Geometry check sheet. Reference: the model listing, model coordinates, mm. A direction names the side the tool comes from. Give positions to 0.01 mm unless a question says otherwise; leave off trailing zeros. Loops run counter-clockwise (first coordinate to the right, second up) from the corner with the lowest first, then second, coordinate; pieces in that order, holes last.
1. Cross-section at B-B, the plane y = 0. State how many separate pieces and enclosed holes the cut face has, plus the area to 3 significant figures.
2. Material ranges on L1, parallel to Y at x = 7.5, z = 0; L2, parallel to X at y = 0, z = 2.6; L3, parallel to Y at x = 17.25, z = 0, recorded low to high.
3. Cross-section at A-A, the plane x = 16.5. Record the cut outline in (y, z), plus the area to 3 significant figures.
4. Tool access check on faces 1 (the cylindrical face through (16.7, -3.6, 2.8)), 2 (the conical face through (8.226, 5.081, 5.134)), 3 (the cylindrical face through (10.046, 0.596, 2.919)). Record the directions out of +Z, -Z, +X, -X, +Y, -Y that give a thin tool (end or side, any length) a straight path to the whole face; none if there is none.
5. Go/stop test with flat-tipped pins: pin 1 Ø1 at (y, z) = (-4, -2.5) entering from +X; pin 2 Ø3 at (x, z) = (3.5, 2) entering from +Y. Record where each tip stops, or that it passes through.
from build123d import *

# Parameters (mm, degrees)
SKETCH3_W          = 1.5748
SKETCH3_H          = 4.5593
HOLE1_D            = 3.2512
HOLE1_DEPTH        = 21.463
HOLE1_CSINK_D      = 4.0132
HOLE1_CSINK_ANGLE  = 90
SKETCH6_W          = 25.4
SKETCH6_H          = 25.4
SKETCH6_W_2        = 12.7
SKETCH6_H_2        = 12.7
CUT_EXTRUDE1_DEPTH = 21.463
HOLE2_D            = 3.96748
HOLE2_DEPTH        = 6.35
HOLE2_CSINK_D      = 4.826
HOLE2_CSINK_ANGLE  = 90


with BuildPart() as part:
    # Sketch1 → Revolve1 (revolve)
    with BuildSketch(Plane.XY):
        Polygon((0, 0), (0, 4.13258), (0.62992, 4.7625), (7.9248, 4.7625), (7.9248, 0), align=None)
    revolve(axis=Axis((7.9248, 0, 0), (-1, 0, 0)))

    # Sketch2 → Revolve2 (revolve)
    with BuildSketch(Plane.XY):
        Polygon((7.9248, 0), (7.9248, 6.9215), (8.6868, 7.6835), (15.1003, 7.6835), (15.8623, 6.9215), (15.8623, 3.52425), (17.9959, 3.52425), (18.5547, 4.08305), (20.955, 4.08305), (21.463, 3.57505), (21.463, 0), align=None)
    revolve(axis=Axis((21.463, 0, 0), (-1, 0, 0)))

    # Sketch3 → Revolve3 (revolve)
    with BuildSketch(Plane.XY):
        with Locations((16.6497, 2.27965)):
            Rectangle(SKETCH3_W, SKETCH3_H)
    revolve(axis=Axis((17.4371, 0, 0), (-1, 0, 0)))

    # Hole1
    with Locations(Plane.ZY):
        with Locations((0, 0)):
            CounterSinkHole(HOLE1_D / 2, HOLE1_CSINK_D / 2, depth=HOLE1_DEPTH, counter_sink_angle=HOLE1_CSINK_ANGLE)

    # Sketch6 → Cut-Extrude1 (cut)
    with BuildSketch(Plane(origin=(0, 0, 0), x_dir=(0, 0, -1), z_dir=(1, 0, 0))):
        Rectangle(SKETCH6_W, SKETCH6_H)
        Rectangle(SKETCH6_W_2, SKETCH6_H_2, mode=Mode.SUBTRACT)
    extrude(amount=CUT_EXTRUDE1_DEPTH, mode=Mode.SUBTRACT)

    # Hole2
    with Locations(Plane.XY.offset(6.35)):
        with Locations((11.938, 0)):
            CounterSinkHole(HOLE2_D / 2, HOLE2_CSINK_D / 2, depth=HOLE2_DEPTH, counter_sink_angle=HOLE2_CSINK_ANGLE)

    # Sketch9 → Revolve4 (revolve)
    with BuildSketch(Plane.XY):
        with BuildLine():
            Line((17.4371, 3.27025), (17.9959, 3.27025))
            Line((17.9959, 3.27025), (17.9959, 3.52425))
            Line((17.9959, 3.52425), (17.7165, 3.52425))
            Line((17.7165, 3.52425), (17.550871292, 3.689878708))
            ThreePointArc((17.550871292, 3.689878708), (17.513673853, 3.779681269), (17.550871292, 3.869483831))
            Line((17.550871292, 3.869483831), (18.156519265, 4.475131804))
            Line((18.156519265, 4.475131804), (18.156519265, 4.5593))
            Line((18.156519265, 4.5593), (17.953319265, 4.5593))
            Line((17.953319265, 4.5593), (17.4371, 4.043080735))
            Line((17.4371, 4.043080735), (17.4371, 3.27025))
        make_face()
    revolve(axis=Axis((17.9959, 0, 0), (-1, 0, 0)))


solid = part.part
Result:
1. separate pieces: 3
1. enclosed holes: 0
1. area: 134 mm2
2. L1: y = -4.76 to -1.63, 1.63 to 4.76
2. L2: x = 0 to 9.95, 13.92 to 21.46
2. L3: y = -4.56 to -1.63, 1.63 to 4.56
3. outline: circle Ø9.12 at (0, 0); hole circle Ø3.25 at (0, 0)
3. area: 57.0 mm2
4. face 1: +X
4. face 2: +Z, -X, +Y
4. face 3: +Z
5. pin 1: stops at x = 18.16
5. pin 2: stops at y = 4.74
